Input: part model. Units: mm. Frame: model coordinates. A direction names the side the tool comes from. Give positions to 0.01 mm unless a question says otherwise; leave off trailing zeros. Order: outer loops, then holes, each group sorted by start corner. A loop starts at its lowest first (then second) coordinate and runs counter-clockwise, first axis right, second up. Notation, with made-up numbers: (-12.75, 42) - (-2.75, 42) arc R9 ccw to (-2.75, 55) - close; hole circle Ø11 at (-11.75, 85). An arc over 180 degrees is marked (long way). Answer in a Markdown table with one row per item. Add a question column.
from build123d import *

# Parameters (mm, degrees)
F0_R     = 5.75
F1_DEPTH = 12.5
F1_TAPER = -3
F3_DEPTH = 11
F4_R     = 1.5


with BuildPart() as f1:
    # F0 (on Top) → F1 (new body)
    with BuildSketch(Plane.XY):
        Circle(F0_R)
    extrude(amount=F1_DEPTH, taper=F1_TAPER)

    # F2 (on face) → F3 (cut)
    with BuildSketch(Plane.XY.offset(12.5)):
        with BuildLine():
            Line((-4.8323294905, -9.4099955732), (-1.494225813, -4.1916332401))
            ThreePointArc((-1.494225813, -4.1916332401), (2.3979489295, 3.7486452128), (-3.1790101783, -3.1139033842))
            Line((-3.1790101783, -3.1139033842), (-6.5171138558, -8.3322657173))
            Line((-6.5171138558, -8.3322657173), (-4.8323294905, -9.4099955732))
        make_face()
    extrude(amount=-F3_DEPTH, mode=Mode.SUBTRACT)

    # F4
    f4_edges = [f1.edges().sort_by_distance(p)[0] for p in [
        (-5.75, 0, 0),
    ]]
    fillet(f4_edges, radius=F4_R)


solid = f1.part
Q1. Pull-direction query (X, two-part tool) for faces 3 (the flat face through (-1.5, 4.4, 12.5)), 4 (the conical face through (-4.86, -3.72, 7.04)), 5 (the flat face through (0, 0, 1.5)), 6 (the flat face through (-3.589, -3.754, 7.077)); classes: +X half, -X half, draft (parallel to the pull), parting line (faces both ways), or undercut.
Q2. Line query: probe 1 along Z at (x, y) = (-3.75, 0); probe 2 along Y at (x, z) = (0, 8); probe 3 along Y at (x, z) = (0, 4.75). Output: solid intervals per line, ascending.
Q3. Contact query for flat-ended pins moving along their axis: P1, Ø1, axis at x = -2, z = 9.5, coming from the +Y side; P2, Ø1.5, axis at x = 3.5, z = 6.5, coming from the -Y side; P3, Ø1, axis at x = 5, z = 9.5, coming from the +Y side. Output: stop coordinate, or through.
Q4. Section C-C, the plane z = 3.25. Return loops of the section in (x, y).
Q5. Section A-A, the plane x = 0. Return loops of the section in (y, z), then the cut area to 3 significant figures.
Q6. Access query for faces 1 (the flat face through (0, 0, 0)), 2 (the flat face through (-1.92, -4.86, 7.08)). Directions: +Z, -Z, +X, -X, +Y, -Y. A direction counts if a zero-diameter tool reaches every point of the face in a straight line with its end or side. Return the directions, or none.
Q7. Section B-B, the plane z = 9.25. Return loops of the section in (x, y), then the cut area to 3 significant figures.
Computed:
| question | item | result |
|---|---|---|
| 1 | face 3 | draft |
| 1 | face 4 | parting line |
| 1 | face 5 | undercut |
| 1 | face 6 | undercut |
| 2 | probe 1 | z = 0 to 1.5 |
| 2 | probe 2 | y = -6.17 to -4.45, 4.45 to 6.17 |
| 2 | probe 3 | y = -6 to -4.45, 4.45 to 6 |
| 3 | P1 | stops at y = 6.07 |
| 3 | P2 | stops at y = -5.44 |
| 3 | P3 | stops at y = 4.34 |
| 4 | outline | (-3.99, -4.38) - (-3.18, -3.11) arc R4.45 cw (long way) to (-1.49, -4.19) - (-2.3, -5.45) arc R5.92 ccw (long way) to start |
| 5 | outline | (-6.41, 12.5) - (-5.82, 1.42) arc R1.5 ccw to (-4.33, 0) - (4.33, 0) arc R1.5 ccw to (5.82, 1.42) - (6.41, 12.5) - (4.45, 12.5) - (4.45, 1.5) - (-4.45, 1.5) - (-4.45, 12.5) - close |
| 5 | area | 53.2 mm^2 |
| 6 | face 1 | -Z, +X, -X, +Y, -Y |
| 6 | face 2 | +Z |
| 7 | outline | (-4.16, -4.65) - (-3.18, -3.11) arc R4.45 cw (long way) to (-1.49, -4.19) - (-2.47, -5.72) arc R6.23 ccw (long way) to start |
| 7 | area | 56.3 mm^2 |
